from build123d import *

# Parameters (mm, degrees)
SKETCH4_W           = 176.492
SKETCH4_H           = 129.883
BOSS_EXTRUDE1_DEPTH = 25
SKETCH5_OUTSIDE_W   = 222.602
SKETCH5_OUTSIDE_H   = 175.993
SKETCH5_OUTSIDE_W_2 = 176.492
SKETCH5_OUTSIDE_H_2 = 129.883
SKETCH5_OUTSIDE_W_3 = 166.492
SKETCH5_OUTSIDE_H_3 = 119.883
CUT_EXTRUDE1_DEPTH  = 20
SKETCH7_W           = 176.492
SKETCH7_H           = 129.883
SKETCH7_W_2         = 171.452
SKETCH7_H_2         = 124.843
CUT_EXTRUDE2_DEPTH  = 10
SKETCH12_R          = 36
CUT_EXTRUDE3_DEPTH  = 15
SKETCH13_R          = 2.5
CUT_EXTRUDE4_DEPTH  = 15
FILLET1_R           = 2


with BuildPart() as part:
    # Sketch4 → Boss-Extrude1 (new body)
    with BuildSketch(Plane.XY.offset(10)):
        with Locations((63.246, 39.9415)):
            Rectangle(SKETCH4_W, SKETCH4_H)
    extrude(amount=BOSS_EXTRUDE1_DEPTH)

    # Sketch5 outside → Cut-Extrude1 (cut)
    with BuildSketch(Plane(origin=(0, 0, 10), x_dir=(-1, 0, 0), z_dir=(0, 0, -1))):
        with Locations((-63.246, 39.9415)):
            Rectangle(SKETCH5_OUTSIDE_W, SKETCH5_OUTSIDE_H)
        with Locations((-63.246, 39.9415)):
            Rectangle(SKETCH5_OUTSIDE_W_2, SKETCH5_OUTSIDE_H_2, mode=Mode.SUBTRACT)
        with Locations((-63.246, 39.9415)):
            Rectangle(SKETCH5_OUTSIDE_W_3, SKETCH5_OUTSIDE_H_3)
    extrude(amount=-CUT_EXTRUDE1_DEPTH, mode=Mode.SUBTRACT)

    # Sketch7 → Cut-Extrude2 (cut)
    with BuildSketch(Plane(origin=(0, 0, 10), x_dir=(-1, 0, 0), z_dir=(0, 0, -1))):
        with Locations((-63.246, 39.9415)):
            Rectangle(SKETCH7_W, SKETCH7_H)
        with Locations((-63.246, 39.9415)):
            Rectangle(SKETCH7_W_2, SKETCH7_H_2, mode=Mode.SUBTRACT)
    extrude(amount=-CUT_EXTRUDE2_DEPTH, mode=Mode.SUBTRACT)

    # Sketch12 → Cut-Extrude3 (cut)
    with BuildSketch(Plane.XY.offset(35)):
        with Locations((63.246, 39.9415)):
            Circle(SKETCH12_R)
    extrude(amount=-CUT_EXTRUDE3_DEPTH, mode=Mode.SUBTRACT)

    # Sketch13 → Cut-Extrude4 (cut)
    with BuildSketch(Plane.XY.offset(35)):
        with Locations((27.246, 75.9415)):
            Circle(SKETCH13_R)
        with Locations((99.246, 75.9415)):
            Circle(SKETCH13_R)
        with Locations((99.246, 3.9415)):
            Circle(SKETCH13_R)
        with Locations((27.246, 3.9415)):
            Circle(SKETCH13_R)
    extrude(amount=-CUT_EXTRUDE4_DEPTH, mode=Mode.SUBTRACT)

    # Fillet1
    fillet1_edges = [part.edges().sort_by_distance(p)[0] for p in [
        (151.492, 39.9415, 35),
        (63.246, 104.883, 35),
        (-25, 39.9415, 35),
        (-25, 104.883, 27.5),
        (151.492, 104.883, 27.5),
        (151.492, -25, 27.5),
        (-25, -25, 27.5),
        (63.246, -25, 35),
    ]]
    fillet(fillet1_edges, radius=FILLET1_R)


solid = part.part
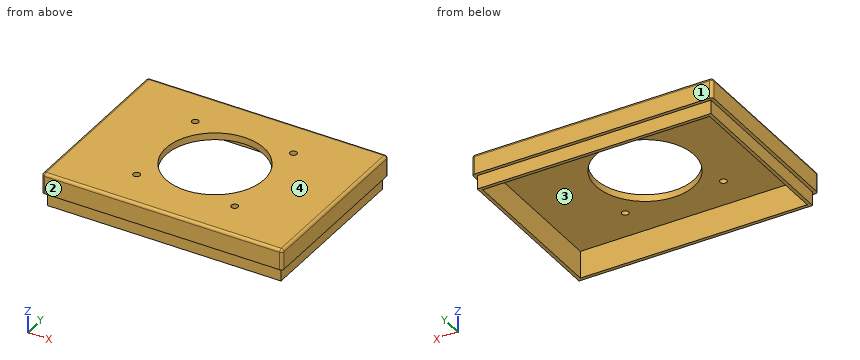
Could you check a few things on this model? Use its own coordinates, in mm. Face numbers are marked on the shaded views. Give positions to 0.01 mm unless a question says otherwise; leave off trailing zeros. Order: outer loops, then holes, each group sorted by start corner. A loop starts at its lowest first (then second) coordinate and runs counter-clockwise, first axis right, second up.
Item 1: If we section it at A-A, the plane z = 17.75: Write out the boundary of the cut face in (x, y).
Item 2: If we section it at C-C, the plane y = 71: Write out the boundary of the cut face in (x, z).
Item 3: If we mould it in two halves opening along Y, with no side actions, what happens to the marked faces 1, 2, 3 and 4? For each: pulls with the +Y half, pulls with the -Y half, needs draft (parallel to the pull), parting line crosses it, or undercut.
Item 4: If we section it at D-D, the plane y = -7.5: Write out the boundary of the cut face in (x, z), plus the area to 3 significant figures.
Item 5: I'm going to push flat-ended pins straight in: pin 1 (8 mm diameter, centred on x = 20.5, z = 13.5, fed in from -Y); pin 2 (4 mm diameter, centred on x = 4.5, y = 49, fed in from -Z); pin 3 (3 mm diameter, centred on x = 99.25, y = 75.94, fed in from +Z); pin 4 (5 mm diameter, centred on x = 43.5, z = 14.5, fed in from +Y). Where does each tip first touch, or does it pass through?
Item 6: I need wall thicknesses on line 1 (X direction, y = 2.5, z = 21); line 2 (X direction, y = 43.5, z = 16); line 3 (Y direction, x = -15.5, z = 16). Which ranges of each line are inside material? Lowest first, please.
Item 7: If we section it at B-B, the plane x = -1: Write out the boundary of the cut face in (y, z).
Values:
1. outline: (-22.48, -22.48) - (148.97, -22.48) - (148.97, 102.36) - (-22.48, 102.36) - close; hole (-20, -20) - (146.49, -20) - (146.49, 99.88) - (-20, 99.88) - close
2. outline: (-25, 20) - (-22.48, 20) - (-22.48, 10) - (-20, 10) - (-20, 30) - (45.04, 30) - (45.04, 35) - (-23, 35) arc R2 ccw to (-25, 33) - close; (81.45, 30) - (146.49, 30) - (146.49, 10) - (148.97, 10) - (148.97, 20) - (151.49, 20) - (151.49, 33) arc R2 ccw to (149.49, 35) - (81.45, 35) - close
3. face 1: pulls with the +Y half
3. face 2: pulls with the -Y half
3. face 3: undercut
3. face 4: needs draft
4. outline: (-25, 20) - (-22.48, 20) - (-22.48, 10) - (-20, 10) - (-20, 30) - (146.49, 30) - (146.49, 10) - (148.97, 10) - (148.97, 20) - (151.49, 20) - (151.49, 33) arc R2 ccw to (149.49, 35) - (-23, 35) arc R2 ccw to (-25, 33) - close
4. area: 1,030 mm2
5. pin 1: stops at y = -22.48
5. pin 2: stops at z = 30
5. pin 3: passes through
5. pin 4: stops at y = 102.36
6. line 1: x = -25 to -20, 146.49 to 151.49
6. line 2: x = -22.48 to -20, 146.49 to 148.97
6. line 3: y = -22.48 to -20, 99.88 to 102.36
7. outline: (-25, 20) - (-22.48, 20) - (-22.48, 10) - (-20, 10) - (-20, 30) - (99.88, 30) - (99.88, 10) - (102.36, 10) - (102.36, 20) - (104.88, 20) - (104.88, 33) arc R2 ccw to (102.88, 35) - (-23, 35) arc R2 ccw to (-25, 33) - close
